Geometry check sheet. Reference: the model listing, model coordinates, mm. Give positions to 0.01 mm unless a question says otherwise; leave off trailing zeros. Write each loop counter-clockwise with the first axis right and the second up, starting at its lowest first coordinate (ties: lowest second). Pieces come first, ordered by that corner, then holes. Notation, with made-up numbers: M 58.5,-16 L 91.5,-16 A33 cw 91.5,14 Z; hole C 3,-9 d1. An arc over 180 degrees is marked long. One line per item, written item: value. Start each with the question number.
1. Scan lines: line 1 (Z direction, x = 0, y = -30.5); line 2 (X direction, y = -37, z = 3.5). Record each from-to range of solid material in increasing order.
2. Cross-section at A-A on y = -46. Record the cut outline in (x, z), then the cut area to 3 significant figures.
3. Gauge pin test, flat ends, axial feed: pin 1 (3 mm diameter, centred on y = -17, z = 2, fed in from +X); pin 2 (6 mm diameter, centred on x = 17, z = 1, fed in from -Y). Record the tip position at first contact, or that the pin passes through.
4. Release check for a two-part mould opening along Z. For faces 1 (the face through (0, -32, 4)), 2 (the face through (0, -48.67, 3.5)), 3 (the face through (9.484, -12.369, 7.184)), 4 (the face through (9.1, -12.5, 0)) record: pulls with the +Z half, pulls with the -Z half, needs draft (parallel to the pull), parting line crosses it, or undercut.
from build123d import *

# Parameters (mm, degrees)
SKETCH6_R = 0.5


with BuildPart() as part:
    # Sweep1: sweep along a curve in space
    with BuildLine() as sweep1_path:
        ThreePointArc((-12, 0, 0), (-8.485281374, -8.485281374, 0), (0, -12, 0))
        Line((0, -12, 0), (18, -12, 0))
        ThreePointArc((18, -12, 0), (23.251188525, -12, 6.434532027), (15.894563339, -12, 10.289171986))
        Line((15.894563339, -12, 10.289171986), (2.988770327, -12, 4.776617378))
        ThreePointArc((2.988770327, -12, 4.776617378), (0.875390561, -12.951902961, 3.873912573), (0, -15.25, 3.5))
        Line((0, -15.25, 3.5), (0, -48.67, 3.5))
    # Sketch6 → Sweep1 (sweep)
    with BuildSketch(Plane(origin=(0, 0, 0), x_dir=(1, 0, 0), z_dir=(0, 1, 0))):
        with Locations((-12, 0)):
            Circle(SKETCH6_R)
    sweep(path=sweep1_path.line)


solid = part.part
Report:
1. line 1: z = 3 to 4
1. line 2: x = -0.5 to 0.5
2. outline: C 0,3.5 d1
2. area: 0.785 mm^2
3. pin 1: stops at x = 0.5
3. pin 2: stops at y = -12.5
4. face 1: parting line crosses it
4. face 2: needs draft
4. face 3: undercut
4. face 4: undercut
